The drawing under review shows one solid part. Ordinate dimensions are in mm from its lowest x, y, z. A direction names the side the tool comes from. Coordinates: 2 decimals unless noted, no trailing zeros. Order: outer loops, then holes, each group sorted by start corner. A loop starts at its lowest first (then second) coordinate and runs counter-clockwise, first axis right, second up.
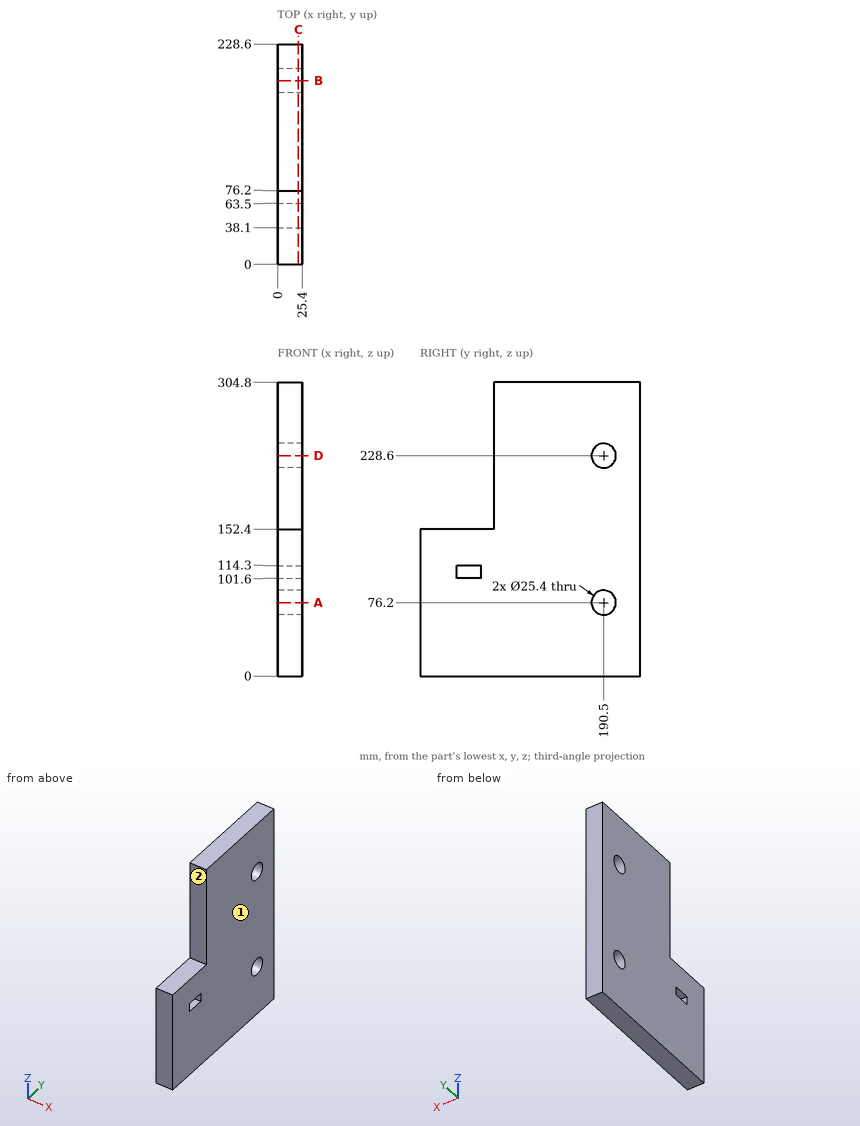
1. Add section A-A (z = 76.2). Give the boundary of the cut face in (x, y), and give its area (3 significant figures).
2. To check wall thickness, follow line 1 (Z direction, x = 14.5, y = 190.5); line 2 (Z direction, x = 13.5, y = 45); line 3 (Z direction, x = 17.75, y = 183). State the ranges of each line that lie inside material, in increasing order.
3. Add section C-C (x = 21.5). Give the boundary of the cut face in (y, z).
4. Add section B-B (y = 190.5). Give the boundary of the cut face in (x, z).
5. For the marked faces 1 and 2, list the 3-axis set-ups (+Z, -Z, +X, -X, +Y, -Y) from which the entire face can be reached by the end or side of a thin tool; tool diameter is ignored.
6. Add section D-D (z = 228.6). Give the boundary of the cut face in (x, y), and give its area (3 significant figures).
7. Insertion check: pin 1 (7.5 mm diameter, centred on x = 17.5, z = 212, fed in from -Y); pin 2 (8 mm diameter, centred on x = 15.5, y = 28.5, fed in from +Z). Each pin has a flat end and moves straight along its axis. Give the tip position at first contact, or say it passes through.
Solution:
1. outline: (0, 0) - (25.4, 0) - (25.4, 177.8) - (0, 177.8) - close; (0, 203.2) - (25.4, 203.2) - (25.4, 228.6) - (0, 228.6) - close
1. area: 5,160 mm2
2. line 1: z = 0 to 63.5, 88.9 to 215.9, 241.3 to 304.8
2. line 2: z = 0 to 101.6, 114.3 to 152.4
2. line 3: z = 0 to 65.95, 86.45 to 218.35, 238.85 to 304.8
3. outline: (0, 0) - (228.6, 0) - (228.6, 304.8) - (76.2, 304.8) - (76.2, 152.4) - (0, 152.4) - close; hole (38.1, 101.6) - (63.5, 101.6) - (63.5, 114.3) - (38.1, 114.3) - close; hole circle Ø25.4 at (190.5, 76.2); hole circle Ø25.4 at (190.5, 228.6)
4. outline: (0, 0) - (25.4, 0) - (25.4, 63.5) - (0, 63.5) - close; (0, 88.9) - (25.4, 88.9) - (25.4, 215.9) - (0, 215.9) - close; (0, 241.3) - (25.4, 241.3) - (25.4, 304.8) - (0, 304.8) - close
5. face 1: +Z, -Z, +X, +Y, -Y
5. face 2: +Z, +X, -X, -Y
6. outline: (0, 76.2) - (25.4, 76.2) - (25.4, 177.8) - (0, 177.8) - close; (0, 203.2) - (25.4, 203.2) - (25.4, 228.6) - (0, 228.6) - close
6. area: 3,230 mm2
7. pin 1: stops at y = 76.2
7. pin 2: stops at z = 152.4
